Here's how the part is built. I have some questions about the finished solid (model axes, mm). A direction names the side the tool comes from. Coordinates: 2 decimals unless noted, no trailing zeros. Write each loop counter-clockwise with the first axis right and the second up, starting at its lowest first coordinate (ties: lowest second). Pieces come first, ordered by that corner, then holes. Notation, with made-up numbers: (-29, 36.5) - (-3, 36.5) arc R22 ccw to (-3, 72.5) - close; hole circle Ø9 at (5, 63.25). An arc over 180 degrees is marked (long way). Answer in a Markdown table with one row per item. Add a question column.
Item 1: I'm going to push flat-ended pins straight in: pin 1 (1 mm diameter, centred on x = 0, z = -4, fed in from -Y); pin 2 (4 mm diameter, centred on x = 5.5, z = 7, fed in from +Y); pin 3 (2 mm diameter, centred on x = -4.5, z = -1, fed in from +Y) (3 decimals). Where does each tip first touch, or does it pass through?
Item 2: Imagine slicing it at A-A (z = -7.75). Please give me the cut outline in (x, y).
Item 3: Imagine slicing it at B-B (y = -7.5). Please give me the cut outline in (x, z), plus the area to 3 significant figures.
Item 4: Which directions (+Z, -Z, +X, -X, +Y, -Y) give clear straight access to the entire face, cutting with the end or side of a thin tool? Please do faces 5 (the face through (22.18, 0.17, 1.26)), 6 (the face through (25.4, 0, 2)), 7 (the face through (0, 5, 9)).
Item 5: Imagine slicing it at C-C (x = 9.5). Please give me the cut outline in (y, z), plus the area to 3 significant figures.
Item 6: We'd pull the mould along Y, two halves only. Please class faces 1 (the face through (31.84, -0.09, -8.75)), 2 (the face through (32, 3.975, 4)), 3 (the face through (-25.4, 0, 0)), 4 (the face through (-12.522, 7.559, -5.796)): +Y half, -Y half, draft (parallel to the pull), parting line (faces both ways), or undercut.
Item 7: Imagine slicing it at D-D (z = -3.5). Please give me the cut outline in (x, y).
Item 8: If I drill on probe 1 along Y at (x, z) = (21.25, 0); probe 2 along X at (y, z) = (-7, -9.5), over which ranges is the centre line in solid material (lowest first)? Write a range as from..to.
from build123d import *

# Parameters (mm, degrees)
F0_R     = 12.7
F1_DEPTH = 25.4
F3_DEPTH = 12.7
F4_R     = 9.525
F5_DEPTH = 25.4
F7_D     = 2.54
F7_DEPTH = 6.35
F7_TIP   = 0.7630929862
F9_DEPTH = 12.7


with BuildPart() as f1:
    # F0 (on Right) → F1 (new body)
    with BuildSketch(Plane.YZ):
        Circle(F0_R)
    extrude(amount=F1_DEPTH)

    # F2 (on face) → F3 (join)
    with BuildSketch(Plane.YZ.offset(25.4)):
        with BuildLine():
            ThreePointArc((3.9751, 0), (0, -3.9751), (-3.9751, 0))
            Line((-3.9751, 0), (-3.9751, 12.0618646979))
            ThreePointArc((-3.9751, 12.0618646979), (0, -12.7), (3.9751, 12.0618646979))
            Line((3.9751, 12.0618646979), (3.9751, 0))
        make_face()
    extrude(amount=F3_DEPTH)

    # F4 (on face) → F5 (join)
    with BuildSketch(Plane(origin=(0, 0, 0), x_dir=(0, -1, 0), z_dir=(-1, 0, 0))):
        Circle(F4_R)
    extrude(amount=F5_DEPTH)

    # F7
    with Locations(Plane.YZ.offset(25.4)):
        with Locations((0, 0)):
            Hole(F7_D / 2, depth=F7_DEPTH)
            with Locations((0, 0, -(F7_DEPTH + F7_TIP / 2))):  # 118° drill point
                Cone(0, F7_D / 2, F7_TIP, mode=Mode.SUBTRACT)


with BuildPart() as f9:
    # F8 (on face) → F9 (new body)
    with BuildSketch(Plane.YZ.offset(38.1)):
        with BuildLine():
            Line((-3.9751, 0), (-3.9751, -4.7752))
            ThreePointArc((-3.9751, -4.7752), (0, -8.7503), (3.9751, -4.7752))
            Line((3.9751, -4.7752), (3.9751, 0))
            ThreePointArc((3.9751, 0), (0, -3.9751), (-3.9751, 0))
        make_face()
    extrude(amount=-F9_DEPTH)


with BuildPart() as f1_1:
    add(f1.part)

    # F10: cut F9
    add(f9.part, mode=Mode.SUBTRACT)


solid = f1_1.part
Here are the results:
| question | item | result |
|---|---|---|
| 1 | pin 1 | stops at y = -12.21 |
| 1 | pin 2 | stops at y = 11.67 |
| 1 | pin 3 | stops at y = 9.525 |
| 2 | outline | (-25.4, -5.54) - (0, -5.54) - (0, -10.06) - (38.1, -10.06) - (38.1, -2.64) - (25.4, -2.64) - (25.4, 2.64) - (38.1, 2.64) - (38.1, 10.06) - (0, 10.06) - (0, 5.54) - (-25.4, 5.54) - close |
| 3 | outline | (-25.4, -5.87) - (0, -5.87) - (0, -10.25) - (38.1, -10.25) - (38.1, 10.25) - (0, 10.25) - (0, 5.87) - (-25.4, 5.87) - close |
| 3 | area | 1,080 mm2 |
| 4 | face 5 | +X |
| 4 | face 6 | +Z, +X |
| 4 | face 7 | -X |
| 5 | outline | circle Ø25.4 at (0, 0) |
| 5 | area | 507 mm2 |
| 6 | face 1 | undercut |
| 6 | face 2 | undercut |
| 6 | face 3 | draft |
| 6 | face 4 | parting line |
| 7 | outline | (-25.4, -8.86) - (0, -8.86) - (0, -12.21) - (38.1, -12.21) - (38.1, -3.98) - (25.4, -3.98) - (25.4, 3.98) - (38.1, 3.98) - (38.1, 12.21) - (0, 12.21) - (0, 8.86) - (-25.4, 8.86) - close |
| 8 | probe 1 | y = -12.7..-1.27, 1.27..12.7 |
| 8 | probe 2 | x = 0..38.1 |
